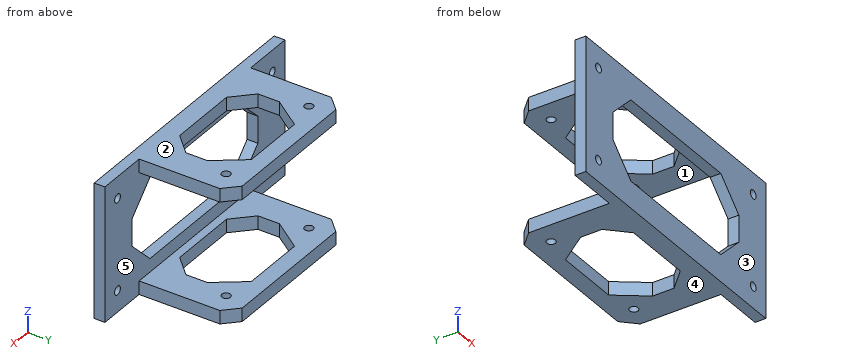
from build123d import *

# Parameters (mm, degrees)
SKETCH_1_W          = 100
SKETCH_1_H          = 50
SKETCH_1_R          = 1.6
EXTRUDE_1_DEPTH     = 4
SKETCH_2_W          = 72
SKETCH_2_H          = 5
EXTRUDE_2_DEPTH     = 35
SKETCH_3_R          = 1.6
CUT_EXTRUDE_1_DEPTH = 51
CUT_EXTRUDE_2_DEPTH = 51
CUT_EXTRUDE_3_DEPTH = 5


with BuildPart() as part:
    # 草图1 → 凸台-拉伸1 (new body)
    with BuildSketch(Plane(origin=(0, 0, 0), x_dir=(1, 0, 0), z_dir=(0, 1, 0))):
        Rectangle(SKETCH_1_W, SKETCH_1_H)
        with Locations((-43, 17)):
            Circle(SKETCH_1_R, mode=Mode.SUBTRACT)
        with Locations((-43, -17)):
            Circle(SKETCH_1_R, mode=Mode.SUBTRACT)
        with Locations((43, -17)):
            Circle(SKETCH_1_R, mode=Mode.SUBTRACT)
        with Locations((43, 17)):
            Circle(SKETCH_1_R, mode=Mode.SUBTRACT)
    extrude(amount=EXTRUDE_1_DEPTH)

    # 草图2 → 凸台-拉伸2 (add)
    with BuildSketch(Plane(origin=(0, 4, 0), x_dir=(1, 0, 0), z_dir=(0, 1, 0))):
        with Locations((0, 22.5)):
            Rectangle(SKETCH_2_W, SKETCH_2_H)
        with Locations((0, -22.5)):
            Rectangle(SKETCH_2_W, SKETCH_2_H)
    extrude(amount=EXTRUDE_2_DEPTH)

    # 草图3 → 切除-拉伸1 (cut, through all)
    with BuildSketch(Plane(origin=(0, 0, -25), x_dir=(-1, 0, 0), z_dir=(0, 0, -1))):
        with Locations((-23, 31)):
            Circle(SKETCH_3_R)
        with Locations((23, 31)):
            Circle(SKETCH_3_R)
        Polygon((-26, 39), (-36, 29), (-36, 39), align=None)
        Polygon((36, 39), (26, 39), (36, 29), align=None)
    extrude(amount=-CUT_EXTRUDE_1_DEPTH, mode=Mode.SUBTRACT)

    # 草图4 → 切除-拉伸2 (cut, through all)
    with BuildSketch(Plane(origin=(0, 0, -25), x_dir=(-1, 0, 0), z_dir=(0, 0, -1))):
        Polygon((12, 33), (-12, 33), (-20, 22.035391732), (-20, 14.035391732), (-13, 7.035391732), (13, 7.035391732), (20, 14.035391732), (20, 22.035391732), align=None)
        Polygon((-36, 4), (-31, 4), (-31, 34), (-36, 29), align=None)
        Polygon((31, 34), (36, 29), (36, 4), (31, 4), align=None)
    extrude(amount=-CUT_EXTRUDE_2_DEPTH, mode=Mode.SUBTRACT)

    # 草图5 → 切除-拉伸3 (cut, through all)
    with BuildSketch(Plane(origin=(0, 4, 0), x_dir=(1, 0, 0), z_dir=(0, 1, 0))):
        Polygon((-25, 15), (-35, 5), (-35, -5), (-25, -15), (25, -15), (35, -5), (35, 5), (25, 15), align=None)
    extrude(amount=-CUT_EXTRUDE_3_DEPTH, mode=Mode.SUBTRACT)


solid = part.part
Could you check a few things on this model? Use its own coordinates, in mm. Face numbers are marked on the shaded views. A direction names the side the tool comes from. Coordinates: 2 decimals unless noted, no trailing zeros. Order: outer loops, then holes, each group sorted by start corner. A loop starts at its lowest first (then second) coordinate and runs counter-clockwise, first axis right, second up.
Q1. Which directions (+Z, -Z, +X, -X, +Y, -Y) give clear straight access to the entire face, cutting with the end or side of a thin tool? Please do the marked faces 1 and 2.
Q2. Suppose I cut it at D-D on z = -17. Please give me the cut outline in (x, y).
Q3. Please list where these lines run through material, in increasing order: L1, parallel to X at y = 1, z = 17; L2, parallel to Z at x = 43, y = 3; L3, parallel to Z at x = -2.5, y = 34.
Q4. Will these pins go through, and if not, where does the flat tip stop? pin 1 (5.5 mm diameter, centred on y = 17.5, z = 23.5, fed in from -X); pin 2 (4 mm diameter, centred on y = 22, z = 23.5, fed in from +X); pin 3 (12 mm diameter, centred on x = 32, z = 2.5, fed in from +Y).
Q5. Suppose I cut it at B-B on x = -8. Please give me the cut outline in (y, z).
Q6. Suppose I cut it at A-A on z = 9.5. Please give me the cut outline in (x, y), and give its area (3 significant figures).
Q7. Thinking about a two-plate mould opening in Z: for the marked faces 3, 4 and 5, which applies, released by +Z, released by -Z, zero draft, split by the parting line, or undercut?
Q8. Suppose I cut it at C-C on y = 5. Please give me the cut outline in (x, z).
Answer:
1. face 1: +X, -X, +Y
1. face 2: +Z, +X, -X, +Y, -Y
2. outline: (-50, 0) - (-44.6, 0) - (-44.6, 4) - (-50, 4) - close; (-41.4, 0) - (41.4, 0) - (41.4, 4) - (-41.4, 4) - close; (44.6, 0) - (50, 0) - (50, 4) - (44.6, 4) - close
3. L1: x = -50 to -44.6, -41.4 to 41.4, 44.6 to 50
3. L2: z = -25 to -18.6, -15.4 to 15.4, 18.6 to 25
3. L3: z = -25 to -20, 20 to 25
4. pin 1: stops at x = -31
4. pin 2: stops at x = 31
4. pin 3: stops at y = 4
5. outline: (0, -25) - (7.04, -25) - (7.04, -20) - (4, -20) - (4, -15) - (0, -15) - close; (0, 15) - (4, 15) - (4, 20) - (7.04, 20) - (7.04, 25) - (0, 25) - close; (33, -25) - (39, -25) - (39, -20) - (33, -20) - close; (33, 20) - (39, 20) - (39, 25) - (33, 25) - close
6. outline: (-50, 0) - (-30.5, 0) - (-30.5, 4) - (-50, 4) - close; (30.5, 0) - (50, 0) - (50, 4) - (30.5, 4) - close
6. area: 156 mm2
7. face 3: zero draft
7. face 4: released by -Z
7. face 5: undercut
8. outline: (-31, -25) - (31, -25) - (31, -20) - (-31, -20) - close; (-31, 20) - (31, 20) - (31, 25) - (-31, 25) - close
